```python
from build123d import *

# Parameters (mm, degrees)
F0_W      = 70
F0_H      = 70
F1_DEPTH  = 2
F3_D      = 2.54
F4_W      = 70
F4_H      = 8
F5_DEPTH  = 11.6
F6_W      = 69.909066
F6_H      = 27
F7_DEPTH  = 3
F8_W      = 20
F8_H      = 7
F9_DEPTH  = 12
F10_W     = 70.34298
F10_H     = 43
F11_DEPTH = 3
F12_W     = 8
F12_H     = 9.2
F13_DEPTH = 4.6


with BuildPart() as f1:
    # F0 (on Top) → F1 (new body)
    with BuildSketch(Plane.XY):
        Rectangle(F0_W, F0_H)
    extrude(amount=F1_DEPTH)

    # F3 (through all)
    with Locations(Plane(origin=(0, 0, 0), x_dir=(1, 0, 0), z_dir=(0, 0, -1))):
        with Locations((-30, 30), (30, 30), (-30, -30), (30, -30)):
            Hole(F3_D / 2)

    # F4 (on face) → F5 (join)
    with BuildSketch(Plane.XY.offset(2)):
        with Locations((0, 18)):
            Rectangle(F4_W, F4_H)
    extrude(amount=F5_DEPTH)

    # F6 (on face) → F7 (join)
    with BuildSketch(Plane.XY.offset(13.6)):
        with Locations((-0.045467, 17.5)):
            Rectangle(F6_W, F6_H)
    extrude(amount=F7_DEPTH)

    # F8 (on face) → F9 (join)
    with BuildSketch(Plane.XY.offset(2)):
        with Locations((0, -31.5)):
            Rectangle(F8_W, F8_H)
    extrude(amount=F9_DEPTH)

    # F10 (on face) → F11 (join)
    with BuildSketch(Plane.XY.offset(14)):
        with Locations((0.205681, -49.460026)):
            Rectangle(F10_W, F10_H)
    extrude(amount=F11_DEPTH)

    # F12 (on face) → F13 (join)
    with BuildSketch(Plane.XY.offset(17)):
        with Locations((-6.465809, -66.360026)):
            Rectangle(F12_W, F12_H)
    extrude(amount=F13_DEPTH)


solid = f1.part
```
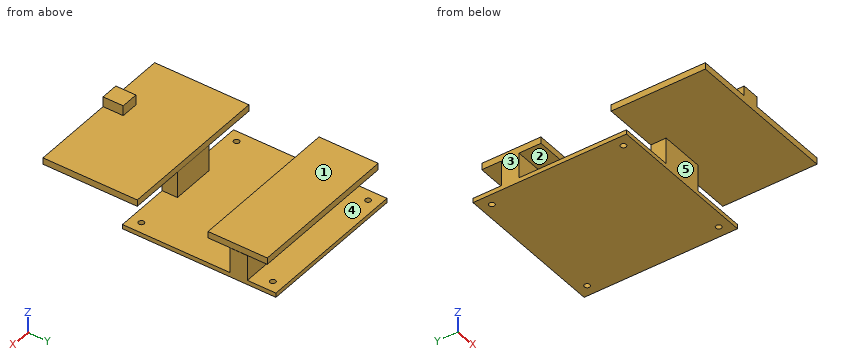
The model under review builds one solid part; all positions refer to its coordinate system, in mm. Face numbers are marked on the shaded views. A direction names the side the tool comes from. Give positions to 0.01 mm unless a question says otherwise; leave off trailing zeros. Write each loop counter-clockwise with the first axis right and the second up, starting at its lowest first coordinate (ties: lowest second). Pieces come first, ordered by that corner, then holes. Notation, with made-up numbers: M -8.75,3.5 L -3.75,3.5 A19 ccw -3.75,38.5 Z; hole C 18.5,80.25 d6. An arc over 180 degrees is marked long. Write each question's results on one line, items separated by ' | '. Start each with the question number.
1. Mouldability with a two-part tool opening along Z and no side actions: class the marked faces 1 and 2 as released by +Z, released by -Z, zero draft, split by the parting line, or undercut.
2. We need section C-C (y = 7). Write out the cut boundary in (x, z).
3. We need section A-A (y = -30). Write out the cut boundary in (x, z), and give its area (3 significant figures).
4. We need section B-B (x = 24). Write out the cut boundary in (y, z), and give its area (3 significant figures).
5. Insertion check: pin 1 Ø4 at (x, z) = (26.5, 4.5) entering from -Y; pin 2 Ø2.5 at (x, z) = (16, 15) entering from +Y; pin 3 Ø2 at (y, z) = (-32.5, 8) entering from -X; pin 4 Ø1 at (x, z) = (-13, 18) entering from -Y. Each pin has a flat end and moves straight along its axis. Give the tip position at first contact, or say it passes through.
6. We need section D-D (z = 8). Write out the cut boundary in (x, y).
7. For probe 1 along X at (y, z) = (-30, 1.5); probe 2 along Z at (x, y) = (26.5, -31), list the stretches that pass through material, from the lowest coordinate up. Write a range as [from, to].
8. For the marked faces 3, 4 and 5, list the 3-axis set-ups (+Z, -Z, +X, -X, +Y, -Y) from which the entire face can be reached by the end or side of a thin tool; tool diameter is ignored.
Results found:
1) face 1: released by +Z | face 2: undercut
2) outline: M -35,0 L 35,0 L 35,2 L -35,2 Z; M -35,13.6 L 34.91,13.6 L 34.91,16.6 L -35,16.6 Z
3) outline: M -35,0 L -31.27,0 L -31.27,2 L -35,2 Z; M -34.97,14 L -10,14 L -10,2 L -28.73,2 L -28.73,0 L 28.73,0 L 28.73,2 L 10,2 L 10,14 L 35.38,14 L 35.38,17 L -34.97,17 Z; M 31.27,0 L 35,0 L 35,2 L 31.27,2 Z | area: 581 mm^2
4) outline: M -70.96,14 L -27.96,14 L -27.96,17 L -70.96,17 Z; M -35,0 L 35,0 L 35,2 L 22,2 L 22,13.6 L 31,13.6 L 31,16.6 L 4,16.6 L 4,13.6 L 14,13.6 L 14,2 L -35,2 Z | area: 443 mm^2
5) pin 1: stops at y = 14 | pin 2: stops at y = 31 | pin 3: stops at x = -10 | pin 4: passes through
6) outline: M -35,14 L 35,14 L 35,22 L -35,22 Z; M -10,-35 L 10,-35 L 10,-28 L -10,-28 Z
7) probe 1: x = [-35, -31.27], [-28.73, 28.73], [31.27, 35] | probe 2: z = [0, 2], [14, 17]
8) face 3: +Z, -Z, -X, +Y, -Y | face 4: +X, -X, +Y | face 5: -Z, +X, -X, -Y
